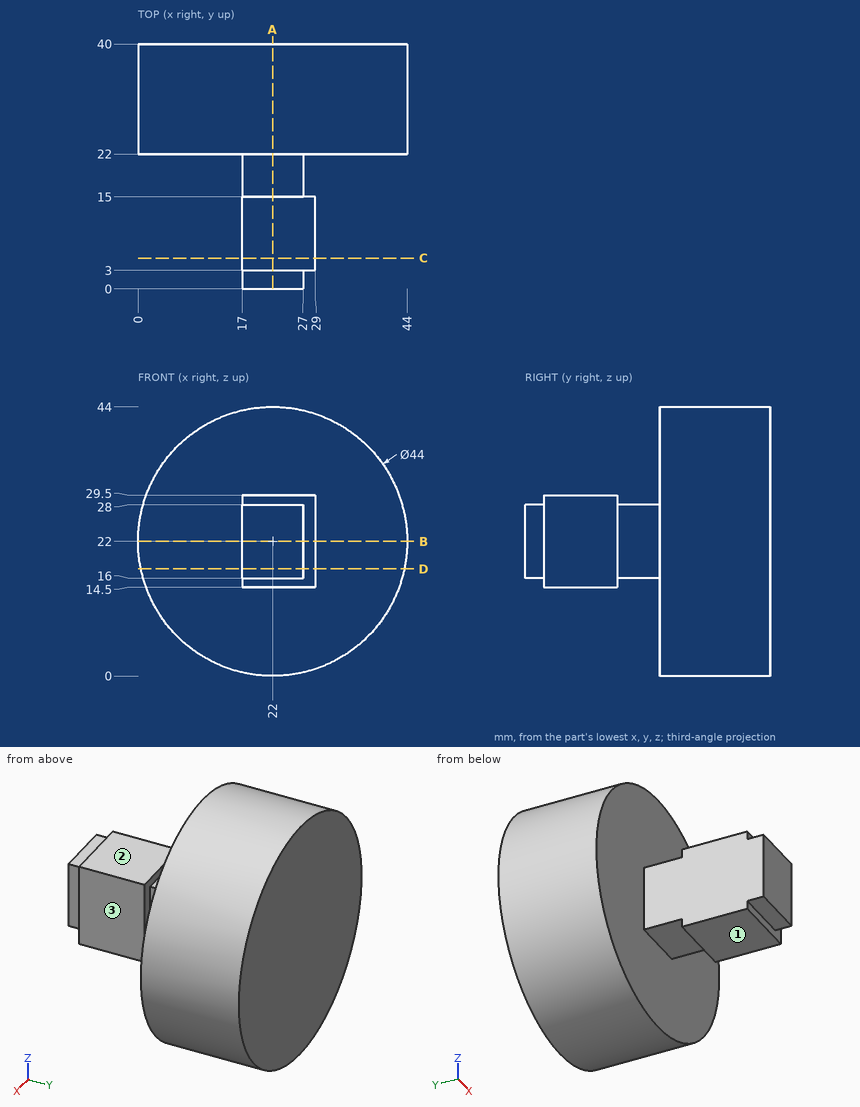
Print and shaded views of the part. All mm, measured from the part's lowest x, y and z. A direction names the side the tool comes from. Coordinates: 2 decimals unless noted, no trailing zeros. Write each loop counter-clockwise with the first axis right and the second up, starting at its lowest first coordinate (ties: lowest second). Pieces come first, ordered by that corner, then holes. Notation, with made-up numbers: (86.25, 54.5) - (112.25, 54.5) arc R10 cw to (112.25, 58.5) - close; hole circle Ø2 at (15, 61.25). An arc over 180 degrees is marked (long way). One line per question, with ' | ' between items. Start each with the question number.
Q1. Cut at D-D, the plane z = 17.5. List the corners of the cut face in (x, y), then the cut area to 3 significant figures.
Q2. Cut at B-B, the plane z = 22. List the corners of the cut face in (x, y), then the cut area to 3 significant figures.
Q3. 3-axis set-ups, long thin cutter, end or side, ignore diameter. For the marked faces 1, 2 and 3: which of +Z, -Z, +X, -X, +Y, -Y reach the whole face in a straight line?
Q4. Drill centre lines: line 1 (Y direction, x = 23, z = 42); line 2 (X direction, y = 12, z = 23.5); line 3 (Z direction, x = 22, y = 21). Where is each one in solid material? Low to high. Write a range as [from, to].
Q5. Pin check, flat tips, straight feed: pin 1 (4 mm diameter, centred on x = 24.5, y = 29.5, fed in from -Z); pin 2 (3.5 mm diameter, centred on x = 21, y = 1, fed in from -Z); pin 3 (3.5 mm diameter, centred on x = 20, y = 1.5, fed in from +Z); pin 4 (3.5 mm diameter, centred on x = 20, z = 21.5, fed in from -Y). Stop position of each tip, or through.
Q6. Cut at C-C, the plane y = 5. List the corners of the cut face in (x, z).
Q7. Cut at A-A, the plane x = 22. List the corners of the cut face in (y, z).
Answer below:
1) outline: (0.47, 22) - (17, 22) - (17, 0) - (27, 0) - (27, 3) - (29, 3) - (29, 15) - (27, 15) - (27, 22) - (43.53, 22) - (43.53, 40) - (0.47, 40) - close | area: 1,020 mm^2
2) outline: (0, 22) - (17, 22) - (17, 0) - (27, 0) - (27, 3) - (29, 3) - (29, 15) - (27, 15) - (27, 22) - (44, 22) - (44, 40) - (0, 40) - close | area: 1,040 mm^2
3) face 1: -Z, +X, -X, -Y | face 2: +Z, +X, -X, -Y | face 3: +Z, -Z, +X, -Y
4) line 1: [22, 40] | line 2: [17, 29] | line 3: [16, 28]
5) pin 1: z = 0.01 | pin 2: z = 16 | pin 3: z = 29.5 | pin 4: y = 0
6) outline: (17, 14.5) - (29, 14.5) - (29, 29.5) - (17, 29.5) - close
7) outline: (0, 16) - (3, 16) - (3, 14.5) - (15, 14.5) - (15, 16) - (22, 16) - (22, 0) - (40, 0) - (40, 44) - (22, 44) - (22, 28) - (15, 28) - (15, 29.5) - (3, 29.5) - (3, 28) - (0, 28) - close
